For this review, take the finished solid that the model builds, in its own axes (mm). Face numbers are marked on the shaded views. A direction names the side the tool comes from. Give positions to 0.01 mm unless a question says otherwise; leave off trailing zeros. Order: outer loops, then holes, each group sorted by start corner. A loop starts at its lowest first (then second) coordinate and runs counter-clockwise, first axis right, second up. Notation, with made-up numbers: (31, -18.5) - (89, -18.5) arc R24 cw to (89, -4.5) - close; hole circle Ø4 at (2.5, -8). An arc over 180 degrees is marked (long way). Use a Markdown table: item, result. Add a question column.
1) Machinability: for the marked faces 4, 5, 6 and 7, which of the approach directions +Z, -Z, +X, -X, +Y, -Y give a long, thin tool a straight path to every point of the face, cutting with its end or side? Answer none if there is none.
2) Wall thickness on L1, parallel to Z at x = 34, y = 21; L2, parallel to Y at x = 4, z = 30.5; L3, parallel to X at y = 65, z = 26: over which ranges is each line inside the solid? List them lowest first.
3) We need section C-C on y = 26. Write out the cut boundary in (x, z).
4) We need section B-B on z = 18.5. Write out the cut boundary in (x, y), then the cut area to 3 significant figures.
5) We need section D-D on x = 26. Write out the cut boundary in (y, z), then the cut area to 3 significant figures.
6) Clearance check with flat-ended pins moving along their axes: P1, Ø5, axis at y = 9.5, z = 30.5, coming from the +X side; P2, Ø12.5, axis at y = 51.5, z = 10, coming from the +X side; P3, Ø21, axis at x = 20, y = 48.5, coming from the +Z side. State where each tip first meets the part, or that it passes through.
7) We need section A-A on z = 28. Write out the cut boundary in (x, y), then the cut area to 3 significant figures.
8) Mouldability with a two-part tool opening along Y and no side actions: class the marked faces 1, 2 and 3 as released by +Y, released by -Y, zero draft, split by the parting line, or undercut.
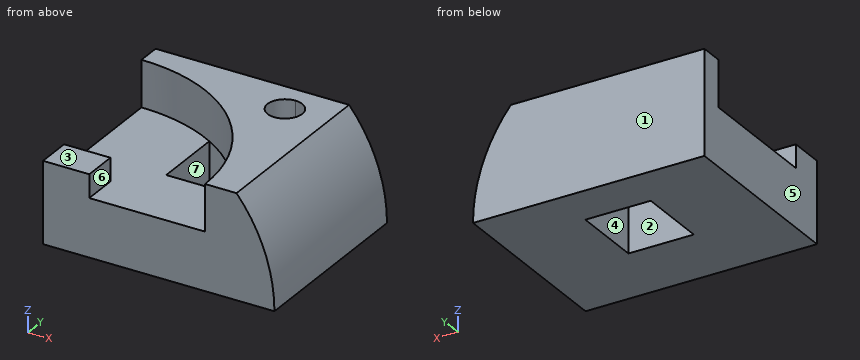
```python
from build123d import *

# Parameters (mm, degrees)
F0_W      = 100
F0_H      = 80
F1_DEPTH  = 45
F3_DEPTH  = 30
F4_R      = 70
F5_DEPTH  = 20
F6_W      = 20
F6_H      = 15
F7_DEPTH  = 10
F9_DEPTH  = 25
F11_DEPTH = 80


with BuildPart() as f1:
    # F0 (on Top) → F1 (new body)
    with BuildSketch(Plane.XY):
        with Locations((50, 40)):
            Rectangle(F0_W, F0_H)
    extrude(amount=F1_DEPTH)

    # F2 (on face) → F3 (cut)
    with BuildSketch(Plane.XY.offset(45)):
        with BuildLine():
            ThreePointArc((72.5, 65), (70.303301, 70.303301), (65, 72.5))
            ThreePointArc((65, 72.5), (59.696699, 59.696699), (72.5, 65))
        make_face()
    extrude(amount=-F3_DEPTH, mode=Mode.SUBTRACT)

    # F4 (on face) → F5 (cut)
    with BuildSketch(Plane.XY.offset(45)):
        Circle(F4_R)
    extrude(amount=-F5_DEPTH, mode=Mode.SUBTRACT)

    # F6 (on face) → F7 (join)
    with BuildSketch(Plane.XY.offset(25)):
        with Locations((10, 7.5)):
            Rectangle(F6_W, F6_H)
    extrude(amount=F7_DEPTH)

    # F8 (on face) → F9 (cut, through all)
    with BuildSketch(Plane.XY.offset(25)):
        Polygon((35, 60.621778), (35, 30), (63.245553, 30), (63.245553, 60.622), align=None)
    extrude(amount=-F9_DEPTH, mode=Mode.SUBTRACT)

    # F10 (on face) → F11 (cut, through all)
    with BuildSketch(Plane.XZ):
        with BuildLine():
            ThreePointArc((83.619026, 45), (95.777397, 23.944395), (100, 0))
            Line((100, 0), (100, 45))
            Line((100, 45), (83.619026, 45))
        make_face()
    extrude(amount=-F11_DEPTH, mode=Mode.SUBTRACT)


solid = f1.part
```
Checked values:
| question | item | result |
|---|---|---|
| 1 | face 4 | -Z |
| 1 | face 5 | +Z, -Z, -X, +Y, -Y |
| 1 | face 6 | +Z, -Y |
| 1 | face 7 | +Z, -Z |
| 2 | L1 | 0 to 25 |
| 2 | L2 | 0 to 15, 69.89 to 80 |
| 2 | L3 | 25.98 to 57.5, 72.5 to 94.99 |
| 3 | outline | (0, 0) - (100, 0) arc R70 ccw to (83.62, 45) - (64.99, 45) - (64.99, 25) - (0, 25) - close |
| 4 | outline | (0, 0) - (97.51, 0) - (97.51, 80) - (0, 80) - close; hole (35, 30) - (63.25, 30) - (63.25, 57.71) arc R7.5 ccw (long way) to (58.91, 60.62) - (35, 60.62) - close |
| 4 | area | 6,770 mm² |
| 5 | outline | (0, 0) - (80, 0) - (80, 45) - (64.99, 45) - (64.99, 25) - (0, 25) - close |
| 5 | area | 2,300 mm² |
| 6 | P1 | x = 94.16 |
| 6 | P2 | x = 99.9 |
| 6 | P3 | z = 25 |
| 7 | outline | (0, 0) - (20, 0) - (20, 15) - (0, 15) - close; (0, 70) arc R70 cw to (70, 0) - (94.16, 0) - (94.16, 80) - (0, 80) - close; hole circle Ø15 at (65, 65) |
| 7 | area | 3,810 mm² |
| 8 | face 1 | released by +Y |
| 8 | face 2 | undercut |
| 8 | face 3 | zero draft |
